from build123d import *

# Parameters (mm, degrees)
F0_R     = 2.54
F1_DEPTH = 7.9375


with BuildPart() as f1:
    # F0 (on Top) → F1 (new body)
    with BuildSketch(Plane.XY):
        with BuildLine():
            Line((47.625, 0), (0, 0))
            Line((0, 0), (0, -1.42875))
            ThreePointArc((0, -1.42875), (1.796051, -2.172699), (2.54, -3.96875))
            ThreePointArc((2.54, -3.96875), (1.796051, -5.764801), (0, -6.50875))
            Line((0, -6.50875), (0, -7.9375))
            Line((0, -7.9375), (47.625, -7.9375))
            Line((47.625, -7.9375), (47.625, -6.50875))
            ThreePointArc((47.625, -6.50875), (45.085, -3.96875), (47.625, -1.42875))
            Line((47.625, -1.42875), (47.625, 0))
        make_face()
        with Locations((7.9375, -3.96875)):
            Circle(F0_R, mode=Mode.SUBTRACT)
        with Locations((15.875, -3.96875)):
            Circle(F0_R, mode=Mode.SUBTRACT)
        with Locations((23.8125, -3.96875)):
            Circle(F0_R, mode=Mode.SUBTRACT)
        with Locations((31.75, -3.96875)):
            Circle(F0_R, mode=Mode.SUBTRACT)
        with Locations((39.6875, -3.96875)):
            Circle(F0_R, mode=Mode.SUBTRACT)
        with BuildLine():
            Line((0, -1.42875), (0, 0))
            ThreePointArc((0, 0), (-3.96875, -3.96875), (0, -7.9375))
            Line((0, -7.9375), (0, -6.50875))
            ThreePointArc((0, -6.50875), (-2.54, -3.96875), (0, -1.42875))
        make_face()
        with BuildLine():
            ThreePointArc((47.625, -7.9375), (51.59375, -3.96875), (47.625, 0))
            Line((47.625, 0), (47.625, -1.42875))
            ThreePointArc((47.625, -1.42875), (49.421051, -2.172699), (50.165, -3.96875))
            ThreePointArc((50.165, -3.96875), (49.421051, -5.764801), (47.625, -6.50875))
            Line((47.625, -6.50875), (47.625, -7.9375))
        make_face()
    extrude(amount=F1_DEPTH)


solid = f1.part
Check sheet for the modelled part. Datum: model origin and axes. Units: mm. Give positions to 0.01 mm unless a question says otherwise; leave off trailing zeros. Loops run counter-clockwise (first coordinate to the right, second up) from the corner with the lowest first, then second, coordinate; pieces in that order, holes last. Notation, with made-up numbers: M 56,11.25 L 65,11.25 A15 cw 65,30.25 Z; hole C 6,-27.5 d1. An arc over 180 degrees is marked long. Use a Markdown table: item, result. Add a question column.
Q1. Go/stop test with flat-tipped pins: pin 1 (1 mm diameter, centred on x = 35.5, z = 1, fed in from +Y); pin 2 (4 mm diameter, centred on x = 31.75, y = -3.97, fed in from +Z); pin 3 (1.5 mm diameter, centred on y = -2, z = 7, fed in from +X). Record where each tip stops, or that it passes through.
Q2. Sectioned sample at D-D, the plane x = 25.5. Record the cut outline in (y, z), then the cut area to 3 significant figures.
Q3. Scan lines: line 1 along Y through (x, z) = (31.75, 3.25); line 2 along Y through (x, z) = (-1, 0.5); line 3 along X through (y, z) = (-7.5, 5.5). Record each from-to range of solid material in increasing order. Write a range as [from, to].
Q4. Mould release check, pull along X, two halves, no side actions. Record for faces 1 (the flat face through (24, 0, 4)), 2 (the cylindrical face through (10.36, -3.21, 3.91)), 3 (the cylindrical face through (-3.968, -3.881, 3.913)): pulls with the +X half, pulls with the -X half, needs draft (parallel to the pull), parting line crosses it, or undercut.
Q5. Sectioned sample at A-A, the plane x = 31.75. Record the cut outline in (y, z).
Q6. Sectioned sample at B-B, the plane z = 2.25. Give the number of separate pieces and of enclosed holes in the cut face, then the cut area to 3 significant figures.
Verdict:
| question | item | result |
|---|---|---|
| 1 | pin 1 | y = 0 |
| 1 | pin 2 | through |
| 1 | pin 3 | x = 51.4 |
| 2 | outline | M -7.94,0 L -5.87,0 L -5.87,7.94 L -7.94,7.94 Z; M -2.07,0 L 0,0 L 0,7.94 L -2.07,7.94 Z |
| 2 | area | 32.9 mm^2 |
| 3 | line 1 | [-7.94, -6.51], [-1.43, 0] |
| 3 | line 2 | [-7.81, -6.3], [-1.63, -0.13] |
| 3 | line 3 | [-1.81, 49.44] |
| 4 | face 1 | needs draft |
| 4 | face 2 | undercut |
| 4 | face 3 | pulls with the -X half |
| 5 | outline | M -7.94,0 L -6.51,0 L -6.51,7.94 L -7.94,7.94 Z; M -1.43,0 L 0,0 L 0,7.94 L -1.43,7.94 Z |
| 6 | separate pieces | 1 |
| 6 | enclosed holes | 7 |
| 6 | area | 286 mm^2 |
